```python
from build123d import *

# Parameters (mm, degrees)
F0_W     = 14
F0_H     = 3
F0_W_2   = 3
F1_DEPTH = 20
F2_DEPTH = 3
F3_W     = 3
F3_H     = 3
F4_DEPTH = 100
F5_W     = 3
F5_H     = 3.5
F6_DEPTH = 100
F7_R     = 1.5
F9_DEPTH = 1


with BuildPart() as f1:
    # F0 (on Front) → F1 (new body)
    with BuildSketch(Plane.XZ):
        Polygon((10, 1.5), (10, 4.5), (-10, 4.5), (-10, 1.5), (-7, 1.5), (7, 1.5), align=None)
        Rectangle(F0_W, F0_H)
        with Locations((11.5, 0)):
            Rectangle(F0_W_2, F0_H)
        with Locations((8.5, 0)):
            Rectangle(F0_W_2, F0_H)
        with Locations((-8.5, 0)):
            Rectangle(F0_W_2, F0_H)
        Polygon((10, -4.5), (10, -1.5), (7, -1.5), (-7, -1.5), (-10, -1.5), (-10, -4.5), align=None)
    extrude(amount=-F1_DEPTH)

    # F0 (on Front) → F2 (join)
    with BuildSketch(Plane.XZ):
        with Locations((-8.5, 0)):
            Rectangle(F0_W_2, F0_H)
        Rectangle(F0_W, F0_H)
        with Locations((8.5, 0)):
            Rectangle(F0_W_2, F0_H)
        with Locations((11.5, 0)):
            Rectangle(F0_W_2, F0_H)
    extrude(amount=F2_DEPTH)

    # F3 (on face) → F4 (cut)
    with BuildSketch(Plane.YZ.offset(13)):
        Polygon((23, -1.75), (23, 1.75), (17, 1.75), (17, 1.5), (20, 1.5), (20, -1.5), (17, -1.5), (17, -1.75), align=None)
        with Locations((18.5, 0)):
            Rectangle(F3_W, F3_H)
    extrude(amount=-F4_DEPTH, mode=Mode.SUBTRACT)

    # F5 (on face) → F6 (cut)
    with BuildSketch(Plane(origin=(0, 17, 0), x_dir=(-1, 0, 0), z_dir=(0, 1, 0))):
        with Locations((11.5, 0)):
            Rectangle(F5_W, F5_H)
        with Locations((8.5, 0)):
            Rectangle(F5_W, F5_H)
    extrude(amount=-F6_DEPTH, mode=Mode.SUBTRACT)

    # F7
    f7_edges = [f1.edges().sort_by_distance(p)[0] for p in [
        (-7, -3, 0),
        (13, -3, 0),
        (10, 0, 3),
        (10, 0, -3),
        (-10, 0, -3.125),
        (-10, 0, 3.125),
        (-7, 17, 0),
        (-10, 20, 3.125),
        (-10, 20, -3.125),
        (13, 17, 0),
        (10, 20, 3.125),
        (10, 20, -3.125),
    ]]
    fillet(f7_edges, radius=F7_R)

    # F8 (on face) → F9 (cut)
    with BuildSketch(Plane.XY.offset(4.5)):
        with BuildLine():
            Line((-1.3400688011, 3), (2.4562410374, 3))
            add(Edge.make_bspline(
                [(5.4571746599, 4.6603732639), (4.2976318515, 3.403944212), (2.4562410374, 3)],
                knots=[0, 0, 0, 0.6784981919, 0.6784981919, 0.6784981919], degree=2))
            add(Edge.make_bspline(
                [(7.1661590349, 9.9605034722), (7.1661590349, 6.5121527778), (5.4571746599, 4.6603732639)],
                knots=[0, 0, 0, 1, 1, 1], degree=2))
            add(Edge.make_bspline(
                [(5.4708465349, 15.2575954861), (7.1661590349, 13.4149305556), (7.1661590349, 9.9605034722)],
                knots=[0, 0, 0, 1, 1, 1], degree=2))
            add(Edge.make_bspline(
                [(0.5763152849, 17.1002604167), (3.7755340349, 17.1002604167), (5.4708465349, 15.2575954861)],
                knots=[0, 0, 0, 1, 1, 1], degree=2))
            add(Edge.make_bspline(
                [(-4.3364451318, 15.2727864583), (-2.6229034651, 17.1002604167), (0.5763152849, 17.1002604167)],
                knots=[0, 0, 0, 1, 1, 1], degree=2))
            add(Edge.make_bspline(
                [(-6.0499867985, 9.9787326389), (-6.0499867985, 13.4453125), (-4.3364451318, 15.2727864583)],
                knots=[0, 0, 0, 1, 1, 1], degree=2))
            add(Edge.make_bspline(
                [(-4.3410024235, 4.6603732639), (-6.0499867985, 6.5121527778), (-6.0499867985, 9.9787326389)],
                knots=[0, 0, 0, 1, 1, 1], degree=2))
            add(Edge.make_bspline(
                [(-1.3400688011, 3), (-3.1814596151, 3.403944212), (-4.3410024235, 4.6603732639)],
                knots=[0.3215018081, 0.3215018081, 0.3215018081, 1, 1, 1], degree=2))
        make_face()
        with BuildLine():
            add(Edge.make_bspline(
                [(-2.9631812429, 9.9605034722), (-2.9631812429, 7.6332465278), (-2.0805857568, 6.4559461806)],
                knots=[0, 0, 0, 1, 1, 1], degree=2))
            add(Edge.make_bspline(
                [(-2.0714711735, 13.4665798611), (-2.9631812429, 12.2847222222), (-2.9631812429, 9.9605034722)],
                knots=[0, 0, 0, 1, 1, 1], degree=2))
            add(Edge.make_bspline(
                [(0.5763152849, 14.6484375), (-1.179761104, 14.6484375), (-2.0714711735, 13.4665798611)],
                knots=[0, 0, 0, 1, 1, 1], degree=2))
            add(Edge.make_bspline(
                [(4.0793534793, 9.9605034722), (4.0793534793, 14.6484375), (0.5763152849, 14.6484375)],
                knots=[0, 0, 0, 1, 1, 1], degree=2))
            add(Edge.make_bspline(
                [(0.5580861182, 5.2786458333), (4.0793534793, 5.2786458333), (4.0793534793, 9.9605034722)],
                knots=[0, 0, 0, 1, 1, 1], degree=2))
            add(Edge.make_bspline(
                [(-2.0805857568, 6.4559461806), (-1.1979902707, 5.2786458333), (0.5580861182, 5.2786458333)],
                knots=[0, 0, 0, 1, 1, 1], degree=2))
        make_face(mode=Mode.SUBTRACT)
    extrude(amount=-F9_DEPTH, mode=Mode.SUBTRACT)


solid = f1.part
```
For this review, take the finished solid that the model builds, in its own axes (mm). A direction names the side the tool comes from. Round coordinates to 2 decimals unless told otherwise and drop trailing zeros. Loops run counter-clockwise (first coordinate to the right, second up) from the corner with the lowest first, then second, coordinate; pieces in that order, holes last.
Q1. Add section A-A on x = -7.5. Write out the cut boundary in (y, z).
Result sheet:
outline: (0, -4.5) - (20, -4.5) - (20, -1.75) - (0, -1.75) - close; (0, 1.75) - (20, 1.75) - (20, 4.5) - (0, 4.5) - close
Q2. To check wall thickness, follow line 1 along Y through (x, z) = (7.5, -2); line 2 along X through (y, z) = (8, 1.25); line 3 along X through (y, z) = (8.5, 2.5). State the ranges of each line that lie inside material, in increasing order.
Result sheet:
line 1: y = 0 to 20
line 2: x = -7 to 13
line 3: x = -10 to 10
Q3. Machinability: for faces 1 (the face through (9.57, 0.45, -2.98)), 2 (the face through (3, 17, 0)), 3 (the face through (6.8, -0.4, 1.5)), which of the approach directions +Z, -Z, +X, -X, +Y, -Y give a long, thin tool a straight path to every point of the face, cutting with its end or side? Answer none if there is none.
Result sheet:
face 1: -Z, +X, -Y
face 2: +X, -X, +Y
face 3: +Z, +X, -Y
Q4. Add section B-B on z = -1. Write out the cut boundary in (x, y).
Result sheet:
outline: (-7, -1.5) arc R1.5 ccw to (-5.5, -3) - (11.5, -3) arc R1.5 ccw to (13, -1.5) - (13, 15.5) arc R1.5 ccw to (11.5, 17) - (-5.5, 17) arc R1.5 ccw to (-7, 15.5) - close
Q5. Insertion check: pin 1 Ø1.8 at (x, z) = (1.5, 0) entering from +Y; pin 2 Ø1 at (x, z) = (-2, -3) entering from -Y; pin 3 Ø1.8 at (y, z) = (9, -0.5) entering from -X. Each pin has a flat end and moves straight along its axis. Give the tip position at first contact, or say it passes through.
Result sheet:
pin 1: stops at y = 17
pin 2: stops at y = 0
pin 3: stops at x = -7
